Input: part model. Units: mm. Frame: model coordinates. A direction names the side the tool comes from. Give positions to 0.01 mm unless a question says otherwise; leave off trailing zeros. Order: outer loops, then holes, each group sorted by start corner. A loop starts at its lowest first (then second) coordinate and runs counter-clockwise, first axis right, second up. Notation, with made-up numbers: (39.25, 83.5) - (85.25, 83.5) arc R30 ccw to (85.25, 117.5) - close; hole circle Ø7 at (-37.75, 86). An arc over 180 degrees is marked (long way). Answer in a Markdown table with one row per item. Add a question column.
1. Access query for faces 1 (the face through (-27, 26, 51.978)), 2 (the face through (-15, 15, 8.874)). Directions: +Z, -Z, +X, -X, +Y, -Y. A direction counts if a zero-diameter tool reaches every point of the face in a straight line with its end or side. Return the directions, or none.
2. Contact query for flat-ended pins moving along their axis: pin 1 (1.5 mm diameter, centred on y = 13.5, z = 43, fed in from -X); pin 2 (1.5 mm diameter, centred on x = -7.5, y = 32, fed in from +Z); pin 3 (1.5 mm diameter, centred on y = 7.5, z = 12.5, fed in from -X). Output: stop coordinate, or through.
3. Section query A-A on z = 14. Return loops of the section in (x, y), and give its area (3 significant figures).
4. Ray query, line 1 (Z direction, x = -31, y = 7.5); line 2 (X direction, y = 16, z = 34); line 3 (X direction, y = 25.5, z = 16). Return the intervals inside material, ascending. Write a range as [from, to].
```python
from build123d import *

# Parameters (mm, degrees)
F1_ANGLE = 90
F2_R     = 5


with BuildPart() as f1:
    # F0 (on Front) → F1 (revolve)
    with BuildSketch(Plane.XZ):
        Polygon((-44.935193, 0), (0, 0), (0, 8.874348), (-36.765158, 8.874348), (-36.765158, 51.978327), (-44.935193, 51.978327), align=None)
    revolve(axis=Axis((0, 0, 4.437174), (0, 0, -1)), revolution_arc=F1_ANGLE)

    # F2
    f2_edges = [f1.edges().sort_by_distance(p)[0] for p in [
        (-31.77398, 31.77398, 51.978327),
        (-31.77398, 31.77398, 0),
    ]]
    fillet(f2_edges, radius=F2_R)


solid = f1.part
```
Answer:
| question | item | result |
|---|---|---|
| 1 | face 1 | +Z, +X, -X, +Y, -Y |
| 1 | face 2 | +Z, +X, -Y |
| 2 | pin 1 | stops at x = -43.09 |
| 2 | pin 2 | stops at z = 8.87 |
| 2 | pin 3 | stops at x = -44.43 |
| 3 | outline | (-44.94, 0) - (-36.77, 0) arc R36.77 cw to (0, 36.77) - (0, 44.94) arc R44.94 ccw to start |
| 3 | area | 524 mm² |
| 4 | line 1 | z = [0, 8.87] |
| 4 | line 2 | x = [-41.99, -33.1] |
| 4 | line 3 | x = [-37, -26.48] |
